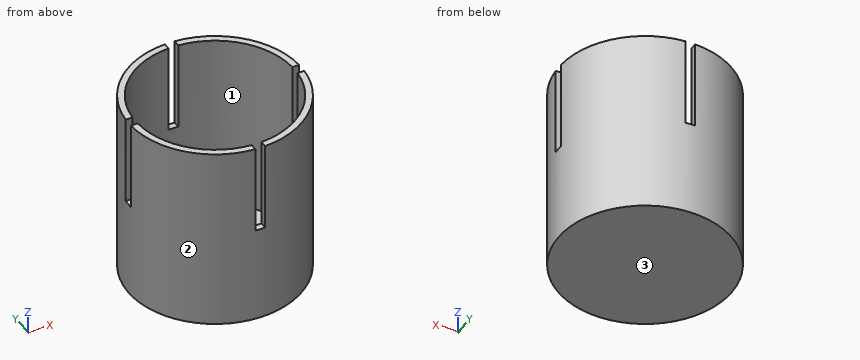
from build123d import *

# Parameters (mm, degrees)
SKETCH_1_R               = 11.5
SKETCH_1_R_2             = 10.6
EXTRUDE_1_DEPTH          = 25
SKETCH_2_R               = 11.5
EXTRUDE_2_DEPTH          = 1
SKETCH_3_W               = 3
SKETCH_3_H               = 1.3
CUT_EXTRUDE_4_DEPTH      = 12
PATTERN_CIRCULAR_1_COUNT = 4


with BuildPart() as part:
    # ｽｹｯﾁ1 → ﾎﾞｽ - 押し出し1 (new body)
    with BuildSketch(Plane.XY):
        Circle(SKETCH_1_R)
        Circle(SKETCH_1_R_2, mode=Mode.SUBTRACT)
    extrude(amount=EXTRUDE_1_DEPTH)

    # ｽｹｯﾁ2 → ﾎﾞｽ - 押し出し2 (add)
    with BuildSketch(Plane.XY):
        Circle(SKETCH_2_R)
    extrude(amount=EXTRUDE_2_DEPTH)

    # ｽｹｯﾁ3 → ｶｯﾄ - 押し出し4 (cut)
    with BuildSketch(Plane.XY.offset(25)):
        with Locations((11.5, 0)):
            Rectangle(SKETCH_3_W, SKETCH_3_H)
    cut_extrude_4 = extrude(amount=-CUT_EXTRUDE_4_DEPTH, mode=Mode.SUBTRACT)

    # 円形ﾊﾟﾀｰﾝ1: ｶｯﾄ - 押し出し4 ×4 about axis
    pattern_circular_1_axis = Axis((0, 0, 0), (0, 0, 1))
    for i in range(1, PATTERN_CIRCULAR_1_COUNT):
        add(cut_extrude_4.rotate(pattern_circular_1_axis, i * 360 / PATTERN_CIRCULAR_1_COUNT), mode=Mode.SUBTRACT)


solid = part.part
Could you check a few things on this model? Use its own coordinates, in mm. Face numbers are marked on the shaded views. Coordinates: 2 decimals unless noted, no trailing zeros. Order: outer loops, then holes, each group sorted by start corner. A loop starts at its lowest first (then second) coordinate and runs counter-clockwise, first axis right, second up.
Q1. Suppose I cut it at D-D on z = 2.5. Please give me the cut outline in (x, y), and give its area (3 significant figures).
Q2. Suppose I cut it at B-B on x = 0. Please give me the cut outline in (y, z).
Q3. Will these pins go through, and if not, where does the flat tip stop? pin 1 (0.7 mm diameter, centred on y = 11, z = 17.5, fed in from -X); pin 2 (0.7 mm diameter, centred on y = -11, z = 17.5, fed in from +X); pin 3 (0.5 mm diameter, centred on x = 0, y = 11, fed in from +Z).
Q4. Thinking about a two-plate mould opening in Y: for the marked faces 1, 2 and 3, which applies, released by +Y, released by -Y, zero draft, split by the parting line, or undercut?
Q5. Please list where these lines run through material, in increasing order: L1, parallel to X at y = -0.5, z = 10; L2, parallel to Y at x = -0.25, z = 2; L3, parallel to Z at x = 6.5, y = -5.
Q6. Suppose I cut it at A-A on z = 15.5. Please give me the cut outline in (x, y), and give its area (3 significant figures).
Answer:
1. outline: circle Ø23 at (0, 0); hole circle Ø21.2 at (0, 0)
1. area: 62.5 mm2
2. outline: (-11.5, 0) - (11.5, 0) - (11.5, 13) - (10.6, 13) - (10.6, 1) - (-10.6, 1) - (-10.6, 13) - (-11.5, 13) - close
3. pin 1: stops at x = -4.34
3. pin 2: stops at x = 4.34
3. pin 3: stops at z = 13
4. face 1: undercut
4. face 2: split by the parting line
4. face 3: zero draft
5. L1: x = -11.49 to -10.59, 10.59 to 11.49
5. L2: y = -11.5 to -10.6, 10.6 to 11.5
5. L3: z = 0 to 1
6. outline: (-11.48, -0.65) arc R11.5 ccw to (-0.65, -11.48) - (-0.65, -10.58) arc R10.6 cw to (-10.58, -0.65) - close; (-11.48, 0.65) - (-10.58, 0.65) arc R10.6 cw to (-0.65, 10.58) - (-0.65, 11.48) arc R11.5 ccw to start; (0.65, -11.48) arc R11.5 ccw to (11.48, -0.65) - (10.58, -0.65) arc R10.6 cw to (0.65, -10.58) - close; (0.65, 10.58) arc R10.6 cw to (10.58, 0.65) - (11.48, 0.65) arc R11.5 ccw to (0.65, 11.48) - close
6. area: 57.8 mm2
